from build123d import *

# Parameters (mm, degrees)
SKETCH1_W               = 80
SKETCH1_H               = 60
BOSS_EXTRUDE1_DEPTH     = 2.5
CUT_EXTRUDE4_DEPTH      = 51.062460986
CUT_EXTRUDE4_DEPTH_BACK = 51.062460986
SKETCH2_R               = 1.6
SKETCH3_W               = 2.5
SKETCH3_H               = 20.5
BOSS_EXTRUDE2_DEPTH     = 66.5
SKETCH4_W               = 80
SKETCH4_H               = 5.5
BOSS_EXTRUDE3_DEPTH     = 2.5
SKETCH5_W               = 2.5
SKETCH5_H               = 5.5
BOSS_EXTRUDE4_DEPTH     = 66.5
SKETCH6_W               = 2.5
SKETCH6_H               = 5.5
CUT_EXTRUDE5_DEPTH      = 66.5
SKETCH9_W               = 2.5
SKETCH9_H               = 2.5
BOSS_EXTRUDE5_DEPTH     = 66.5
SKETCH11_R              = 4.75
CUT_EXTRUDE6_DEPTH      = 2.5
SKETCH15_W              = 2.5
SKETCH15_H              = 23
BOSS_EXTRUDE6_DEPTH     = 8
SKETCH17_W              = 2.5
SKETCH17_H              = 74.5
BOSS_EXTRUDE7_DEPTH     = 2
SKETCH18_R              = 1.6
CUT_EXTRUDE7_DEPTH      = 2.5
SKETCH21_W              = 80
SKETCH21_H              = 2.5
BOSS_EXTRUDE8_DEPTH     = 2
SKETCH22_W              = 4.25
SKETCH22_H              = 74.5
CUT_EXTRUDE8_DEPTH      = 2.5
FILLET1_R               = 5
SKETCH23_W              = 15.225
SKETCH23_H              = 67.5
BOSS_EXTRUDE10_DEPTH    = 2.5
SKETCH24_W              = 95.225
SKETCH24_H              = 10
CUT_EXTRUDE9_DEPTH      = 101.031498164
SKETCH26_W              = 2.5
SKETCH26_H              = 20.75
BOSS_EXTRUDE11_DEPTH    = 74.5
SKETCH27_R              = 1.6
CUT_EXTRUDE10_DEPTH     = 2.5
SKETCH28_W              = 2.5
SKETCH28_H              = 20.75
CUT_EXTRUDE11_DEPTH     = 74.5
SKETCH29_W              = 20.75
SKETCH29_H              = 19.625
CUT_EXTRUDE12_DEPTH     = 2.5
FILLET2_R               = 6
SKETCH31_W              = 13.325
SKETCH31_H              = 57.5
CUT_EXTRUDE13_DEPTH     = 2.5
SKETCH33_W              = 3
SKETCH33_H              = 57.5
CUT_EXTRUDE14_DEPTH     = 2.5
CUT_EXTRUDE15_DEPTH     = 2.5


with BuildPart() as part:
    # Sketch1 → Boss-Extrude1 (new body)
    with BuildSketch(Plane(origin=(0, 0, 0), x_dir=(1, 0, 0), z_dir=(0, 1, 0))):
        Rectangle(SKETCH1_W, SKETCH1_H)
    extrude(amount=BOSS_EXTRUDE1_DEPTH)

    # Sketch2 → Cut-Extrude4 (cut, two sides: drawn at the far end of the back side and taken through both)
    with BuildSketch(Plane(origin=(0, 0, 0), x_dir=(1, 0, 0), z_dir=(0, 1, 0)).offset(-CUT_EXTRUDE4_DEPTH_BACK)):
        with BuildLine():
            Line((-6.25, -24), (-2.5, -24))
            ThreePointArc((-2.5, -24), (0, -21.5), (2.5, -24))
            Line((2.5, -24), (16.25, -24))
            Line((16.25, -24), (16.25, -18))
            Line((16.25, -18), (-6.25, -18))
            Line((-6.25, -18), (-6.25, -24))
        make_face()
        with BuildLine():
            Line((0, -26.5), (0, -30))
            Line((0, -30), (16.25, -30))
            Line((16.25, -30), (16.25, -24))
            Line((16.25, -24), (2.5, -24))
            ThreePointArc((2.5, -24), (1.767766953, -25.767766953), (0, -26.5))
        make_face()
        with BuildLine():
            ThreePointArc((-2.5, -24), (-1.767766953, -25.767766953), (0, -26.5))
            Line((0, -26.5), (0, -24))
            Line((0, -24), (-2.5, -24))
        make_face()
        with BuildLine():
            Line((0, -24), (0, -26.5))
            ThreePointArc((0, -26.5), (1.767766953, -25.767766953), (2.5, -24))
            Line((2.5, -24), (0, -24))
        make_face()
        with BuildLine():
            Line((-2.5, -24), (0, -24))
            Line((0, -24), (2.5, -24))
            ThreePointArc((2.5, -24), (0, -21.5), (-2.5, -24))
        make_face()
        with BuildLine():
            ThreePointArc((-2.5, -24), (-1.767766953, -25.767766953), (0, -26.5))
            Line((0, -26.5), (0, -24))
            Line((0, -24), (-2.5, -24))
        make_face()
        with BuildLine():
            Line((0, -24), (0, -26.5))
            ThreePointArc((0, -26.5), (1.767766953, -25.767766953), (2.5, -24))
            Line((2.5, -24), (0, -24))
        make_face()
        with BuildLine():
            Line((-6.25, -30), (0, -30))
            Line((0, -30), (0, -26.5))
            ThreePointArc((0, -26.5), (-1.767766953, -25.767766953), (-2.5, -24))
            Line((-2.5, -24), (-6.25, -24))
            Line((-6.25, -24), (-6.25, -30))
        make_face()
        with Locations(Location((-8.625, -24, 0), (0, 0, 270))):
            Circle(SKETCH2_R)
        with Locations(Location((18.625, -24, 0), (0, 0, 270))):
            Circle(SKETCH2_R)
    extrude(amount=CUT_EXTRUDE4_DEPTH + CUT_EXTRUDE4_DEPTH_BACK, mode=Mode.SUBTRACT)

    # Sketch3 → Boss-Extrude2 (add)
    with BuildSketch(Plane(origin=(0, 2.5, 0), x_dir=(1, 0, 0), z_dir=(0, 1, 0))):
        with Locations((-38.75, -19.75)):
            Rectangle(SKETCH3_W, SKETCH3_H)
    extrude(amount=BOSS_EXTRUDE2_DEPTH)

    # Sketch4 → Boss-Extrude3 (add)
    with BuildSketch(Plane(origin=(0, 2.5, 0), x_dir=(1, 0, 0), z_dir=(0, 1, 0))):
        with Locations((0, -32.75)):
            Rectangle(SKETCH4_W, SKETCH4_H)
    extrude(amount=-BOSS_EXTRUDE3_DEPTH)

    # Sketch5 → Boss-Extrude4 (add)
    with BuildSketch(Plane(origin=(0, 2.5, 0), x_dir=(1, 0, 0), z_dir=(0, 1, 0))):
        with Locations((-38.75, -32.75)):
            Rectangle(SKETCH5_W, SKETCH5_H)
    extrude(amount=BOSS_EXTRUDE4_DEPTH)

    # Sketch6 → Cut-Extrude5 (cut)
    with BuildSketch(Plane(origin=(0, 69, 0), x_dir=(1, 0, 0), z_dir=(0, 1, 0))):
        with Locations((-38.75, -12.25)):
            Rectangle(SKETCH6_W, SKETCH6_H)
    extrude(amount=-CUT_EXTRUDE5_DEPTH, mode=Mode.SUBTRACT)

    # Sketch9 → Boss-Extrude5 (add)
    with BuildSketch(Plane(origin=(0, 2.5, 0), x_dir=(1, 0, 0), z_dir=(0, 1, 0))):
        with Locations((-38.75, -13.75)):
            Rectangle(SKETCH9_W, SKETCH9_H)
    extrude(amount=BOSS_EXTRUDE5_DEPTH)

    # Sketch11 → Cut-Extrude6 (cut)
    with BuildSketch(Plane(origin=(-37.5, 0, 0), x_dir=(0, 0, -1), z_dir=(1, 0, 0))):
        with Locations((-24, 54)):
            Circle(SKETCH11_R)
    extrude(amount=-CUT_EXTRUDE6_DEPTH, mode=Mode.SUBTRACT)

    # Sketch15 → Boss-Extrude6 (add)
    with BuildSketch(Plane(origin=(0, 69, 0), x_dir=(1, 0, 0), z_dir=(0, 1, 0))):
        with Locations((-38.75, -24)):
            Rectangle(SKETCH15_W, SKETCH15_H)
    extrude(amount=BOSS_EXTRUDE6_DEPTH)

    # Sketch17 → Boss-Extrude7 (add)
    with BuildSketch(Plane.XY.offset(35.5)):
        with Locations((-38.75, 39.75)):
            Rectangle(SKETCH17_W, SKETCH17_H)
    extrude(amount=BOSS_EXTRUDE7_DEPTH)

    # Sketch18 → Cut-Extrude7 (cut)
    with BuildSketch(Plane.ZY.offset(40)):
        with Locations((32, 36.5)):
            Circle(SKETCH18_R)
        with Locations((32, 71.5)):
            Circle(SKETCH18_R)
    extrude(amount=-CUT_EXTRUDE7_DEPTH, mode=Mode.SUBTRACT)

    # Sketch21 → Boss-Extrude8 (add)
    with BuildSketch(Plane.XY.offset(35.5)):
        with Locations((0, 1.25)):
            Rectangle(SKETCH21_W, SKETCH21_H)
    extrude(amount=BOSS_EXTRUDE8_DEPTH)

    # Sketch22 → Cut-Extrude8 (cut)
    with BuildSketch(Plane(origin=(-37.5, 0, 0), x_dir=(0, 0, -1), z_dir=(1, 0, 0))):
        with Locations((-14.625, 39.75)):
            Rectangle(SKETCH22_W, SKETCH22_H)
    extrude(amount=-CUT_EXTRUDE8_DEPTH, mode=Mode.SUBTRACT)

    # Fillet1
    fillet1_edges = [part.edges().sort_by_distance(p)[0] for p in [
        (-38.75, 77, 37.5),
        (-38.75, 77, 16.75),
    ]]
    fillet(fillet1_edges, radius=FILLET1_R)

    # Sketch23 → Boss-Extrude10 (add)
    with BuildSketch(Plane(origin=(0, 2.5, 0), x_dir=(1, 0, 0), z_dir=(0, 1, 0))):
        with Locations((47.6125, -3.75)):
            Rectangle(SKETCH23_W, SKETCH23_H)
    extrude(amount=-BOSS_EXTRUDE10_DEPTH)

    # Sketch24 → Cut-Extrude9 (cut, through all)
    with BuildSketch(Plane(origin=(0, 2.5, 0), x_dir=(1, 0, 0), z_dir=(0, 1, 0))):
        with Locations((7.6125, 25)):
            Rectangle(SKETCH24_W, SKETCH24_H)
    extrude(amount=-CUT_EXTRUDE9_DEPTH, mode=Mode.SUBTRACT)

    # Sketch26 → Boss-Extrude11 (add)
    with BuildSketch(Plane(origin=(0, 2.5, 0), x_dir=(1, 0, 0), z_dir=(0, 1, 0))):
        with Locations((-25.425, -27.125)):
            Rectangle(SKETCH26_W, SKETCH26_H)
    extrude(amount=BOSS_EXTRUDE11_DEPTH)

    # Sketch27 → Cut-Extrude10 (cut)
    with BuildSketch(Plane(origin=(-24.175, 0, 0), x_dir=(0, 0, -1), z_dir=(1, 0, 0))):
        with BuildLine():
            ThreePointArc((-28.75, 36.275), (-27.358757211, 32.916242789), (-24, 31.525))
            Line((-24, 31.525), (-24, 36.275))
            Line((-24, 36.275), (-28.75, 36.275))
        make_face()
        with BuildLine():
            Line((-24, 36.275), (-24, 31.525))
            ThreePointArc((-24, 31.525), (-20.641242789, 32.916242789), (-19.25, 36.275))
            ThreePointArc((-19.25, 36.275), (-24, 41.025), (-28.75, 36.275))
            Line((-28.75, 36.275), (-24, 36.275))
        make_face()
        with BuildLine():
            ThreePointArc((-28.75, 36.275), (-27.358757211, 32.916242789), (-24, 31.525))
            Line((-24, 31.525), (-24, 36.275))
            Line((-24, 36.275), (-28.75, 36.275))
        make_face()
        with BuildLine():
            Line((-24, 36.275), (-24, 31.525))
            ThreePointArc((-24, 31.525), (-20.641242789, 32.916242789), (-19.25, 36.275))
            ThreePointArc((-19.25, 36.275), (-24, 41.025), (-28.75, 36.275))
            Line((-28.75, 36.275), (-24, 36.275))
        make_face()
        with Locations((-32, 18.775)):
            Circle(SKETCH27_R)
        with Locations((-32, 53.775)):
            Circle(SKETCH27_R)
    extrude(amount=-CUT_EXTRUDE10_DEPTH, mode=Mode.SUBTRACT)

    # Sketch28 → Cut-Extrude11 (cut)
    with BuildSketch(Plane(origin=(0, 77, 0), x_dir=(1, 0, 0), z_dir=(0, 1, 0))):
        with Locations((-38.75, -27.125)):
            Rectangle(SKETCH28_W, SKETCH28_H)
    extrude(amount=-CUT_EXTRUDE11_DEPTH, mode=Mode.SUBTRACT)

    # Sketch29 → Cut-Extrude12 (cut)
    with BuildSketch(Plane(origin=(-24.175, 0, 0), x_dir=(0, 0, -1), z_dir=(1, 0, 0))):
        with Locations((-27.125, 67.1875)):
            Rectangle(SKETCH29_W, SKETCH29_H)
    extrude(amount=-CUT_EXTRUDE12_DEPTH, mode=Mode.SUBTRACT)

    # Fillet2
    fillet2_edges = [part.edges().sort_by_distance(p)[0] for p in [
        (-25.425, 57.375, 37.5),
        (-25.425, 57.375, 16.75),
    ]]
    fillet(fillet2_edges, radius=FILLET2_R)

    # Sketch31 → Cut-Extrude13 (cut)
    with BuildSketch(Plane(origin=(0, 2.5, 0), x_dir=(1, 0, 0), z_dir=(0, 1, 0))):
        with Locations((-33.3375, -8.75)):
            Rectangle(SKETCH31_W, SKETCH31_H)
    extrude(amount=-CUT_EXTRUDE13_DEPTH, mode=Mode.SUBTRACT)

    # Sketch33 → Cut-Extrude14 (cut)
    with BuildSketch(Plane(origin=(0, 2.5, 0), x_dir=(1, 0, 0), z_dir=(0, 1, 0))):
        with Locations((53.725, -8.75)):
            Rectangle(SKETCH33_W, SKETCH33_H)
    extrude(amount=-CUT_EXTRUDE14_DEPTH, mode=Mode.SUBTRACT)

    # Sketch34 → Cut-Extrude15 (cut)
    with BuildSketch(Plane(origin=(0, 2.5, 0), x_dir=(1, 0, 0), z_dir=(0, 1, 0))):
        Polygon((-24.175, -16.75), (-24.175, -24.625), (-19.175, -24.625), (-19.175, -22.125), (-16.675, -22.125), (-16.675, -32.125), (-19.175, -32.125), (-19.175, -29.625), (-24.175, -29.625), (-24.175, -37.5), (52.225, -37.5), (52.225, 20), (-26.675, 20), (-26.675, -16.75), align=None)
    extrude(amount=-CUT_EXTRUDE15_DEPTH, mode=Mode.SUBTRACT)


solid = part.part
Could you check a few things on this model? Use its own coordinates, in mm. A direction names the side the tool comes from. Give positions to 0.01 mm unless a question says otherwise; leave off trailing zeros. Order: outer loops, then holes, each group sorted by start corner. A loop starts at its lowest first (then second) coordinate and runs counter-clockwise, first axis right, second up.
1. For faces 4 (the flat face through (-18, 1, 22.125)), 5 (the flat face through (-18, 1, 32.125)), 6 (the flat face through (-22, 1, 29.625)), which set-ups out of +Z, -Z, +X, -X, +Y, -Y let a thin tool reach every point of the face, with its end or its side?
2. We'd pull the mould along Z, two halves only. Please class faces 1 (the flat face through (-19.175, 1, 31)), 2 (the cylindrical face through (-25.41, 17.8, 33.27)), 3 (the cylindrical face through (-25.44, 55.57, 35.79)): pulls with the +Z half, pulls with the -Z half, needs draft (parallel to the pull), parting line crosses it, or undercut.
3. I need wall thicknesses on L1, parallel to Y at x = -25.1, z = 32 (3 decimals); L2, parallel to Y at x = -24.5, z = 31 (3 decimals); L3, parallel to X at y = 42, z = 26.5 (3 decimals). Which ranges of each line are inside material? Lowest first, please.
4. Suppose I cut it at C-C (z = 26.5). List the corners of the cut face in (x, y) for me (3 decimals), plus the area to 3 significant figures.
5. Suppose I cut it at A-A (x = -24.75). List the corners of the cut face in (y, z) for me (3 decimals), plus the area to 3 significant figures.
6. Suppose I cut it at B-B (y = 18). List the corners of the cut face in (x, z) for me (3 decimals), plus the area to 3 significant figures.
7. Will these pins go through, and if not, where does the flat tip stop? P1, Ø1, axis at x = -21, z = 23.5, coming from the -Y side; P2, Ø2, axis at x = -18, y = 1, coming from the +Z side (3 decimals); P3, Ø3, axis at x = -18, y = 1, coming from the -Z side (3 decimals); P4, Ø2, axis at x = -20.5, y = 0.5, coming from the -Z side (3 decimals).
8. Suppose I cut it at D-D (y = 35). List the corners of the cut face in (x, z) for me (3 decimals), plus the area to 3 significant figures.
Solved:
1. face 4: -Z, +X, +Y, -Y
1. face 5: +Z, +X, +Y, -Y
1. face 6: +Z, +Y, -Y
2. face 1: needs draft
2. face 2: undercut
2. face 3: pulls with the +Z half
3. L1: y = 0 to 17.175, 20.375 to 52.175, 55.375 to 57.354
3. L2: y = 0 to 17.526, 20.024 to 52.526, 55.024 to 57.375
3. L3: x = -26.675 to -24.175
4. outline: (-26.675, 0) - (-16.675, 0) - (-16.675, 2.5) - (-24.175, 2.5) - (-24.175, 32.236) - (-26.675, 32.236) - close; (-26.675, 40.314) - (-24.175, 40.314) - (-24.175, 57.375) - (-26.675, 57.375) - close
4. area: 142 mm2
5. outline: (0, 16.75) - (51.375, 16.75) arc R6 ccw to (57.375, 22.75) - (57.375, 31.5) arc R6 ccw to (51.375, 37.5) - (0, 37.5) - close; hole circle Ø3.2 at (18.775, 32); hole circle Ø9.5 at (36.275, 24); hole circle Ø3.2 at (53.775, 32)
5. area: 1,090 mm2
6. outline: (-26.675, 16.75) - (-24.175, 16.75) - (-24.175, 30.6) - (-26.675, 30.6) - close; (-26.675, 33.4) - (-24.175, 33.4) - (-24.175, 37.5) - (-26.675, 37.5) - close
6. area: 44.9 mm2
7. P1: passes through
7. P2: stops at z = 32.125
7. P3: stops at z = 22.125
7. P4: stops at z = 24.625
8. outline: (-26.675, 16.75) - (-24.175, 16.75) - (-24.175, 19.424) - (-26.675, 19.424) - close; (-26.675, 28.576) - (-24.175, 28.576) - (-24.175, 37.5) - (-26.675, 37.5) - close
8. area: 29.0 mm2
